from build123d import *

# Parameters (mm, degrees)
F0_W      = 457.2
F0_H      = 609.6
F1_DEPTH  = 838.2
F2_W      = 206.756
F2_H      = 127
F3_DEPTH  = 25.4
F3_FACE_W = 206.756
F3_FACE_H = 127
F4_DEPTH  = 177.8


with BuildPart() as f1:
    # F0 (on Top) → F1 (new body)
    with BuildSketch(Plane.XY):
        with Locations((228.6, 304.8)):
            Rectangle(F0_W, F0_H)
    extrude(amount=F1_DEPTH)

    # F2 (on face) → F3 (join)
    with BuildSketch(Plane.XZ):
        with Locations((228.6, 431.8)):
            Rectangle(F2_W, F2_H)
    extrude(amount=F3_DEPTH)

    # F3_face (on face) → F4 (join)
    with BuildSketch(Plane(origin=(228.6, -25.4, 431.8), x_dir=(1, 0, 0), z_dir=(0, -1, 0))):
        Rectangle(F3_FACE_W, F3_FACE_H)
    extrude(amount=F4_DEPTH)


solid = f1.part
The listing builds one solid part. Answer for the finished solid, in the listing's coordinates (mm). A direction names the side the tool comes from. Give positions to 0.01 mm unless a question says otherwise; leave off trailing zeros. Write each loop counter-clockwise with the first axis right and the second up, starting at its lowest first coordinate (ties: lowest second). Pieces come first, ordered by that corner, then holes.
1) Section A-A (x = 202) is taken. Write down the section's boundary in (y, z), and give its area (3 significant figures).
2) Find the intervals of material crossed by L1, parallel to Y at x = 409, z = 230.5; L2, parallel to Z at x = 170, y = -143.5; L3, parallel to X at y = -99.5, z = 462.5, in increasing order.
3) A tool of negligible diameter and unlimited length cuts with its end or side. For faces 1 (the face through (331.978, -100, 431)), 2 (the face through (227, -100, 368.3)), 3 (the face through (457.2, 301, 413)), 4 (the face through (227, -100, 495.3)), 5 (the face through (125.222, -100, 431)), from which of +Z, -Z, +X, -X, +Y, -Y can it reach the whole face along a straight path? Write none if from no direction.
4) Section C-C (y = -39.5) is taken. Write down the section's boundary in (x, z), and give its area (3 significant figures).
5) Section D-D (x = 373) is taken. Write down the section's boundary in (y, z).
6) Section B-B (z = 382) is taken. Write down the section's boundary in (x, y).
Response:
1. outline: (-203.2, 368.3) - (0, 368.3) - (0, 0) - (609.6, 0) - (609.6, 838.2) - (0, 838.2) - (0, 495.3) - (-203.2, 495.3) - close
1. area: 537,000 mm2
2. L1: y = 0 to 609.6
2. L2: z = 368.3 to 495.3
2. L3: x = 125.22 to 331.98
3. face 1: +Z, -Z, +X, -Y
3. face 2: -Z, +X, -X, -Y
3. face 3: +Z, -Z, +X, +Y, -Y
3. face 4: +Z, +X, -X, -Y
3. face 5: +Z, -Z, -X, -Y
4. outline: (125.22, 368.3) - (331.98, 368.3) - (331.98, 495.3) - (125.22, 495.3) - close
4. area: 26,300 mm2
5. outline: (0, 0) - (609.6, 0) - (609.6, 838.2) - (0, 838.2) - close
6. outline: (0, 0) - (125.22, 0) - (125.22, -203.2) - (331.98, -203.2) - (331.98, 0) - (457.2, 0) - (457.2, 609.6) - (0, 609.6) - close
